Geometry: final body of the model. Coordinates: model frame, mm. A direction names the side the tool comes from. Round coordinates to 2 decimals unless told otherwise and drop trailing zeros. Write each loop counter-clockwise with the first axis right and the second up, starting at its lowest first coordinate (ties: lowest second). Pieces come first, ordered by that corner, then holes. Notation, with made-up numbers: (55, 7) - (114, 7) arc R25 cw to (114, 43) - close; hole circle Ø2 at (89.5, 13). An arc over 180 degrees is marked (long way). Use a Markdown table: item, result. Add a question column.
```python
from build123d import *

# Parameters (mm, degrees)
SKETCH_4_W             = 20.1
SKETCH_4_H             = 14
EXTRUDE_3_DEPTH        = 6
SKETCH_5_W             = 12.1
SKETCH_5_H             = 4
CUT_EXTRUDE_1_DEPTH    = 19.24835609
SKETCH_6_W             = 3
SKETCH_6_H             = 14
EXTRUDE_4_DEPTH        = 6
EXTRUDE_START          = -6
EXTRUDE_5_DEPTH        = 2
SKETCH_8_W             = 14
SKETCH_8_H             = 2.5
EXTRUDE_6_DEPTH        = 24
CUT_EXTRUDE_2_DEPTH    = 2
SKETCH_10_R            = 0.9
CUT_EXTRUDE_3_DEPTH    = 37.036821447
FILLET_1_R             = 3
HOLE_WIZARD_M2_2_D     = 1.6
HOLE_WIZARD_M2_2_DEPTH = 6
HOLE_WIZARD_M2_2_TIP   = 0.480688495


with BuildPart() as part:
    # 草图4 → 凸台-拉伸3 (new body)
    with BuildSketch(Plane(origin=(0, 0, 0), x_dir=(1, 0, 0), z_dir=(0, 1, 0))):
        Rectangle(SKETCH_4_W, SKETCH_4_H)
    extrude(amount=EXTRUDE_3_DEPTH)

    # 草图5 → 切除-拉伸1 (cut, through all)
    with BuildSketch(Plane.XY.offset(7)):
        with Locations((0, 4)):
            Rectangle(SKETCH_5_W, SKETCH_5_H)
    extrude(amount=-CUT_EXTRUDE_1_DEPTH, mode=Mode.SUBTRACT)

    # 草图6 → 凸台-拉伸4 (add)
    with BuildSketch(Plane.XZ):
        with Locations((8.55, 0)):
            Rectangle(SKETCH_6_W, SKETCH_6_H)
    extrude(amount=EXTRUDE_4_DEPTH)

    # 草图7 → 凸台-拉伸5 (add)
    with BuildSketch(Plane(origin=(0, 0, -7), x_dir=(-1, 0, 0), z_dir=(0, 0, -1)).offset(EXTRUDE_START)):
        Polygon((-7.05, -6), (0, 0), (-7.05, 0), align=None)
    extrude(amount=EXTRUDE_5_DEPTH)

    # 草图8 → 凸台-拉伸6 (add)
    with BuildSketch(Plane(origin=(10.05, 0, 0), x_dir=(0, 0, -1), z_dir=(1, 0, 0))):
        with Locations((0, -4.75)):
            Rectangle(SKETCH_8_W, SKETCH_8_H)
    extrude(amount=EXTRUDE_6_DEPTH)

    # 草图9 → 切除-拉伸2 (cut)
    with BuildSketch(Plane(origin=(0, -3.5, 0), x_dir=(1, 0, 0), z_dir=(0, 1, 0))):
        Polygon((17.75, 4.3), (17.75, -4.3), (26.35, -4.3), (26.35, 4.3), (25.1, 4.3), (25.1, 7), (19, 7), (19, 4.3), align=None)
    extrude(amount=-CUT_EXTRUDE_2_DEPTH, mode=Mode.SUBTRACT)

    # 草图10 → 切除-拉伸3 (cut, through all)
    with BuildSketch(Plane(origin=(0, -3.5, 0), x_dir=(1, 0, 0), z_dir=(0, 1, 0))):
        with Locations(Location((12.55, 0, 0), (0, 0, 270))):
            Circle(SKETCH_10_R)
        with Locations(Location((31.55, 0, 0), (0, 0, 270))):
            Circle(SKETCH_10_R)
    extrude(amount=-CUT_EXTRUDE_3_DEPTH, mode=Mode.SUBTRACT)

    # 圆角1
    fillet_1_edges = [part.edges().sort_by_distance(p)[0] for p in [
        (34.05, -4.75, 7),
        (34.05, -4.75, -7),
    ]]
    fillet(fillet_1_edges, radius=FILLET_1_R)

    # M2 螺纹孔的螺纹孔钻头2
    with Locations(Plane(origin=(-8.05, 6, 0), x_dir=(0, 0, 1), z_dir=(0, 1, 0))):
        with Locations((0, 0), (0, 16.1)):
            Hole(HOLE_WIZARD_M2_2_D / 2, depth=HOLE_WIZARD_M2_2_DEPTH)
            with Locations((0, 0, -(HOLE_WIZARD_M2_2_DEPTH + HOLE_WIZARD_M2_2_TIP / 2))):  # 118° drill point
                Cone(0, HOLE_WIZARD_M2_2_D / 2, HOLE_WIZARD_M2_2_TIP, mode=Mode.SUBTRACT)


solid = part.part
```
1) Set-up query: faces 1 (the flat face through (10.05, 1, 0)), 2 (the flat face through (4, -2, -1)), 3 (the flat face through (19, -4, -6)). Return all of +Z, -Z, +X, -X, +Y, -Y with unobstructed straight access to the full face (end or side cutting, diameter ignored); none if empty.
2) Section A-A, the plane y = 3. Return the cut outline in (x, z).
3) Section C-C, the plane z = 3.5. Return the cut outline in (x, y), then the cut area to 3 significant figures.
4) Section D-D, the plane x = 12.55. Return the cut outline in (y, z).
5) Pin query (flat end, axial travel): P1, Ø3, axis at x = 2, y = -4, coming from the -Z side; P2, Ø3, axis at x = 23, z = 1, coming from the +Y side; P3, Ø1, axis at y = -4, z = -5.5, coming from the -X side; P4, Ø1, axis at x = 16.5, z = -2, coming from the +Y side. Return the tip coordinate at first contact, or that it passes through.
6) Section B-B, the plane x = -8.05. Return the cut outline in (y, z).
7) Material intervals for L1, parallel to X at y = 3.75, z = -2.75; L2, parallel to X at y = -5.1, z = 0; L3, parallel to Z at x = 8.05, y = 1.7, sorted ascending. Write a range as from..to.
8) Draft query along X for faces 4 (the flat face through (34.05, -5, 0)), 5 (the cylindrical face through (7.27, 2.96, 0.17)), 6 (the flat face through (4, -2, -3)). Return one class per face: released by +X, released by -X, zero draft, split by the parting line, or undercut.
Output values:
| question | item | result |
|---|---|---|
| 1 | face 1 | +Z, -Z, +X, +Y |
| 1 | face 2 | +Z, -X, -Y |
| 1 | face 3 | -Z, +Y |
| 2 | outline | (-10.05, -7) - (-6.05, -7) - (-6.05, 7) - (-10.05, 7) - close; (6.05, -7) - (10.05, -7) - (10.05, 7) - (6.05, 7) - close; hole circle Ø1.6 at (-8.05, 0); hole circle Ø1.6 at (8.05, 0) |
| 3 | outline | (-10.05, 0) - (7.05, 0) - (7.05, -6) - (34.05, -6) - (34.05, -3.5) - (26.35, -3.5) - (26.35, -5.5) - (17.75, -5.5) - (17.75, -3.5) - (10.05, -3.5) - (10.05, 6) - (6.05, 6) - (6.05, 2) - (-6.05, 2) - (-6.05, 6) - (-10.05, 6) - close |
| 3 | area | 133 mm^2 |
| 4 | outline | (-6, -7) - (-3.5, -7) - (-3.5, -0.9) - (-6, -0.9) - close; (-6, 0.9) - (-3.5, 0.9) - (-3.5, 7) - (-6, 7) - close |
| 5 | P1 | passes through |
| 5 | P2 | stops at y = -5.5 |
| 5 | P3 | stops at x = 7.05 |
| 5 | P4 | stops at y = -3.5 |
| 6 | outline | (0, -7) - (6, -7) - (6, -0.8) - (0, -0.8) - close; (0, 0.8) - (6, 0.8) - (6, 7) - (0, 7) - close |
| 7 | L1 | x = -10.05..-6.05, 6.05..10.05 |
| 7 | L2 | x = 7.05..11.65, 13.45..17.75, 26.35..30.65, 32.45..34.05 |
| 7 | L3 | z = -7..-0.8, 0.8..7 |
| 8 | face 4 | released by +X |
| 8 | face 5 | undercut |
| 8 | face 6 | zero draft |
